from build123d import *

# Parameters (mm, degrees)
BOSS_EXTRUDE1_DEPTH = 18.6
SKETCH2_R           = 2
SKETCH2_R_2         = 2.5
CUT_EXTRUDE1_DEPTH  = 10
SKETCH3_R           = 50
SKETCH3_R_2         = 45
CUT_EXTRUDE2_DEPTH  = 60
FILLET1_R           = 5
FILLET2_R           = 5
FILLET3_R           = 2
FILLET4_R           = 2


with BuildPart() as part:
    # Sketch1 → Boss-Extrude1 (new body)
    with BuildSketch(Plane.XY):
        Polygon((90, 5), (90, 0), (60, 0), (60, 41), (30, 41), (30, 0), (0, 0), (0, 5), (25, 5), (25, 46), (65, 46), (65, 5), align=None)
    extrude(amount=BOSS_EXTRUDE1_DEPTH)

    # Sketch2 → Cut-Extrude1 (cut)
    with BuildSketch(Plane(origin=(0, 5, 0), x_dir=(1, 0, 0), z_dir=(0, 1, 0))):
        with Locations((75, -9.3)):
            Circle(SKETCH2_R)
        with Locations((15, -9.3)):
            Circle(SKETCH2_R)
        with Locations((28, -9.3)):
            Circle(SKETCH2_R_2)
        with Locations((62, -9.3)):
            Circle(SKETCH2_R_2)
    extrude(amount=-CUT_EXTRUDE1_DEPTH, mode=Mode.SUBTRACT)

    # Sketch3 → Cut-Extrude2 (cut)
    with BuildSketch(Plane(origin=(0, 46, 0), x_dir=(1, 0, 0), z_dir=(0, 1, 0))):
        with Locations((45, -9.3)):
            Circle(SKETCH3_R)
        with Locations((45, -9.3)):
            Circle(SKETCH3_R_2, mode=Mode.SUBTRACT)
    extrude(amount=-CUT_EXTRUDE2_DEPTH, mode=Mode.SUBTRACT)

    # Fillet1
    fillet1_edges = [part.edges().sort_by_distance(p)[0] for p in [
        (25, 46, 9.3),
    ]]
    fillet(fillet1_edges, radius=FILLET1_R)

    # Fillet2
    fillet2_edges = [part.edges().sort_by_distance(p)[0] for p in [
        (65, 46, 9.3),
    ]]
    fillet(fillet2_edges, radius=FILLET2_R)

    # Fillet3
    fillet3_edges = [part.edges().sort_by_distance(p)[0] for p in [
        (60, 0, 14.7),
        (60, 41, 9.3),
        (30, 41, 9.3),
        (30, 0, 14.7),
    ]]
    fillet(fillet3_edges, radius=FILLET3_R)

    # Fillet4
    fillet4_edges = [part.edges().sort_by_distance(p)[0] for p in [
        (60, 0, 3.9),
        (30, 0, 3.9),
    ]]
    fillet(fillet4_edges, radius=FILLET4_R)


solid = part.part
Can you work these out from the model? Positions are in its coordinate system, mm. A direction names the side the tool comes from. Give positions to 0.01 mm unless a question says otherwise; leave off trailing zeros. Order: outer loops, then holes, each group sorted by start corner. A loop starts at its lowest first (then second) coordinate and runs counter-clockwise, first axis right, second up. Notation, with made-up numbers: (27, 78.5) - (83, 78.5) arc R16 ccw to (83, 93.5) - close; hole circle Ø10 at (-33, 32). An arc over 180 degrees is marked (long way). Write each question's results on one line, items separated by ' | '.
1) Suppose I cut it at A-A, the plane x = 15. Write out the boundary of the cut face in (y, z), then the cut area to 3 significant figures.
Final values:
outline: (0, 0) - (5, 0) - (5, 7.3) - (0, 7.3) - close; (0, 11.3) - (5, 11.3) - (5, 18.6) - (0, 18.6) - close | area: 73.0 mm^2
2) On a 3-axis mill with a long thin cutter (end or side, diameter ignored), from which of +Z, -Z, +X, -X, +Y, -Y can I reach the whole of each face in a straight line? I mean faces 1 (the face through (65, 23, 9)), 2 (the face through (12, 5, 9)), 3 (the face through (60.57, 0.6, 3.95)). Say none if no direction works.
Final values:
face 1: +Z, -Z, +X, +Y | face 2: +Z, -Z, -X, +Y | face 3: +Z, -Z, -Y
3) I'm going to push flat-ended pins straight in: pin 1 Ø9.5 at (y, z) = (16, 6.5) entering from -X; pin 2 Ø6.5 at (x, z) = (15, 9.3) entering from +Y; pin 3 Ø4 at (x, z) = (27.5, 4) entering from +Y. Where does each tip first touch, or does it pass through?
Final values:
pin 1: stops at x = 25 | pin 2: stops at y = 5 | pin 3: stops at y = 45.97
4) Suppose I cut it at D-D, the plane x = 29. Write out the boundary of the cut face in (y, z).
Final values:
outline: (0.27, 0) - (45.9, 0) - (45.9, 18.6) - (0.27, 18.6) - (0.27, 11.59) - (5, 11.59) - (5, 7.01) - (0.27, 7.01) - close
5) Please list where these lines run through material, in increasing order: line 1 along X through (y, z) = (2.2, 9.3); line 2 along X through (y, z) = (24, 7.25); line 3 along Z through (x, y) = (28, 2.45). Write a range as [from, to].
Final values:
line 1: x = [0, 13], [17, 25.5], [64.5, 73], [77, 90] | line 2: x = [25, 30], [60, 65] | line 3: z = [0, 6.8], [11.8, 18.6]
6) Suppose I cut it at B-B, the plane y = 30.5. Write out the boundary of the cut face in (x, z).
Final values:
outline: (25, 0) - (30, 0) - (30, 18.6) - (25, 18.6) - close; (60, 0) - (65, 0) - (65, 18.6) - (60, 18.6) - close
7) If we mould it in two halves opening along X, with no side actions, what happens to faces 4 (the face through (62, 20, 18.6)), 5 (the face through (90, 3, 9)), 6 (the face through (45, 41, 9))? For each: pulls with the +X half, pulls with the -X half, needs draft (parallel to the pull), parting line crosses it, or undercut.
Final values:
face 4: needs draft | face 5: pulls with the +X half | face 6: undercut
8) Suppose I cut it at C-C, the plane z = 12.75. Write out the boundary of the cut face in (x, y).
Final values:
outline: (0.13, 0) - (28, 0) arc R2 ccw to (30, 2) - (30, 39) arc R2 cw to (32, 41) - (58, 41) arc R2 cw to (60, 39) - (60, 2) arc R2 ccw to (62, 0) - (89.87, 0) - (89.87, 5) - (65, 5) - (65, 41) arc R5 ccw to (60, 46) - (30, 46) arc R5 ccw to (25, 41) - (25, 5) - (0.13, 5) - close
